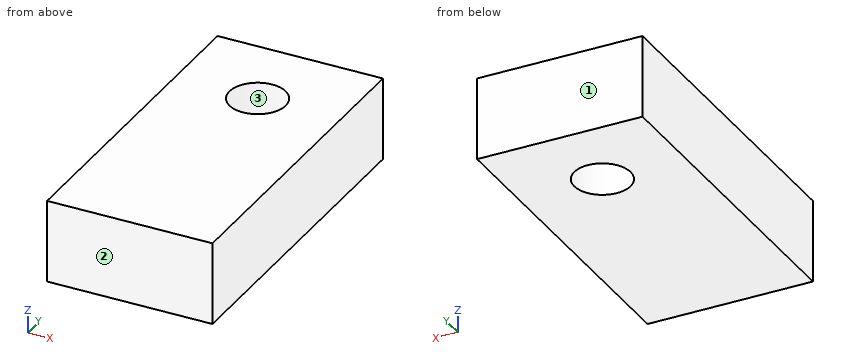
from build123d import *

# Parameters (mm, degrees)
SKETCH1_W               = 30
SKETCH1_H               = 60
BOSS_EXTRUDE1_DEPTH     = 7.5
CUT_EXTRUDE1_DEPTH      = 49.023431781
CUT_EXTRUDE1_DEPTH_BACK = 49.023431781
SKETCH2_R               = 5.1


with BuildPart() as part:
    # Sketch1 → Boss-Extrude1 (new, symmetric)
    with BuildSketch(Plane.XY):
        with Locations((0, -15)):
            Rectangle(SKETCH1_W, SKETCH1_H)
    extrude(amount=BOSS_EXTRUDE1_DEPTH, both=True)

    # Sketch2 → Cut-Extrude1 (cut, two sides: drawn at the far end of the back side and taken through both)
    with BuildSketch(Plane.XY.offset(-CUT_EXTRUDE1_DEPTH_BACK)):
        Circle(SKETCH2_R)
    extrude(amount=CUT_EXTRUDE1_DEPTH + CUT_EXTRUDE1_DEPTH_BACK, mode=Mode.SUBTRACT)


solid = part.part
Could you check a few things on this model? Use its own coordinates, in mm. Face numbers are marked on the shaded views. Give positions to 0.01 mm unless a question says otherwise; leave off trailing zeros. Order: outer loops, then holes, each group sorted by start corner. A loop starts at its lowest first (then second) coordinate and runs counter-clockwise, first axis right, second up.
1. Suppose I cut it at A-A (x = 4.5). List the corners of the cut face in (y, z) for me.
2. I need wall thicknesses on L1, parallel to Y at x = 0, z = 1; L2, parallel to X at y = 0, z = -0.5; L3, parallel to X at y = -2.5, z = -2.5. Which ranges of each line are inside material? Lowest first, please.
3. We'd pull the mould along Y, two halves only. Please class the marked faces 1, 2 and 3: pulls with the +Y half, pulls with the -Y half, needs draft (parallel to the pull), parting line crosses it, or undercut.
4. Suppose I cut it at C-C (z = -3.5). List the corners of the cut face in (x, y) for me, plus the area to 3 significant figures.
5. Suppose I cut it at B-B (y = 0). List the corners of the cut face in (x, z) for me, plus the area to 3 significant figures.
Solved:
1. outline: (-45, -7.5) - (-2.4, -7.5) - (-2.4, 7.5) - (-45, 7.5) - close; (2.4, -7.5) - (15, -7.5) - (15, 7.5) - (2.4, 7.5) - close
2. L1: y = -45 to -5.1, 5.1 to 15
2. L2: x = -15 to -5.1, 5.1 to 15
2. L3: x = -15 to -4.45, 4.45 to 15
3. face 1: pulls with the +Y half
3. face 2: pulls with the -Y half
3. face 3: undercut
4. outline: (-15, -45) - (15, -45) - (15, 15) - (-15, 15) - close; hole circle Ø10.2 at (0, 0)
4. area: 1,720 mm2
5. outline: (-15, -7.5) - (-5.1, -7.5) - (-5.1, 7.5) - (-15, 7.5) - close; (5.1, -7.5) - (15, -7.5) - (15, 7.5) - (5.1, 7.5) - close
5. area: 297 mm2
